```python
from build123d import *

# Parameters (mm, degrees)
FILLET1_R = 7


with BuildPart() as part:
    # Sketch1 → Revolve1 (revolve)
    with BuildSketch(Plane.XY):
        Polygon((25.26151891, 74.539497083), (25.26151891, 61.839497083), (100.628081163, -63.543576688), (104.062419804, -63.543576688), (104.062419804, -64.543576688), (100.062419804, -64.543576688), (24.26151891, 61.562081639), (24.26151891, 74.539497083), (27.567346656, 76.526598412), (27.832759941, 76.085045388), align=None)
    revolve(axis=Axis((0, 0, 0), (0, 1, 0)))

    # Fillet1
    fillet1_edges = [part.edges().sort_by_distance(p)[0] for p in [
        (-25.26151891, 61.839497083, 0),
    ]]
    fillet(fillet1_edges, radius=FILLET1_R)


solid = part.part
```
Source: CAD feature listing. Evaluate the final solid. Frame: model axes, mm. A direction names the side the tool comes from. Give positions to 0.01 mm unless a question says otherwise; leave off trailing zeros. Write each loop counter-clockwise with the first axis right and the second up, starting at its lowest first coordinate (ties: lowest second). Pieces come first, ordered by that corner, then holes. Notation, with made-up numbers: (-34, 20.5) - (6, 20.5) arc R22 ccw to (6, 39.5) - close; hole circle Ø2 at (53.5, -4). An arc over 180 degrees is marked (long way). One line per item, written item: value. Start each with the question number.
Q1. Section query A-A, the plane y = 54.5. Return the cut outline in (x, z), then the cut area to 3 significant figures.
Q2. Section query B-B, the plane y = -23. Return the cut outline in (x, z), then the cut area to 3 significant figures.
Q3. Material intervals for probe 1 along Z at (x, y) = (0, 71); probe 2 along Z at (x, y) = (15, 12.5), sorted ascending. Write a range as from..to.
Q4. First-contact query: pin 1 Ø3 at (x, z) = (45.5, 74) entering from -Y; pin 2 Ø4 at (x, z) = (68, -67) entering from -Y; pin 3 Ø1.5 at (x, y) = (-11, 27) entering from +Z. Flat tips, straight axial feed; report the tip coordinate or a pass-through.
Q5. Set-up query: faces 1 (the face through (54.4, -63.544, -85.3)), 2 (the face through (-82.58, -64.05, 63.32)), 3 (the face through (24.095, 69.085, -7.588)). Return all of +Z, -Z, +X, -X, +Y, -Y with unobstructed straight access to the full face (end or side cutting, diameter ignored); none if empty.
Q6. Draft query along X for faces 4 (the face through (45.25, 24.94, -14.25)), 5 (the face through (-5.304, 74.664, 23.886)), 6 (the face through (-54, -64.544, -85)), 7 (the face through (-19.253, 68.142, 14.763)). Return one class per face: +X half, -X half, draft (parallel to the pull), parting line (faces both ways), or undercut.
Answer:
1. outline: circle Ø59.35 at (0, 0); hole circle Ø57.01 at (0, 0)
1. area: 213 mm2
2. outline: circle Ø152.52 at (0, 0); hole circle Ø150.18 at (0, 0)
2. area: 555 mm2
3. probe 1: z = -25.26..-24.26, 24.26..25.26
3. probe 2: z = -52.83..-51.62, 51.62..52.83
4. pin 1: stops at y = -45.09
4. pin 2: stops at y = -60.22
4. pin 3: stops at z = 45.37
5. face 1: +Y
5. face 2: +Y, -Y
5. face 3: none
6. face 4: parting line
6. face 5: undercut
6. face 6: draft
6. face 7: undercut
